The listing builds one solid part. Answer for the finished solid, in the listing's coordinates (mm). Round coordinates to 2 decimals unless told otherwise and drop trailing zeros. Write each loop counter-clockwise with the first axis right and the second up, starting at its lowest first coordinate (ties: lowest second). Pieces come first, ordered by that corner, then holes. Notation, with made-up numbers: (-31, 67) - (24, 67) arc R7 cw to (24, 71) - close; hole circle Ø6 at (-27, 74.25). An arc over 180 degrees is marked (long way). Answer in a Markdown table with one row per item.
from build123d import *

# Parameters (mm, degrees)
SKETCH1_W           = 210
SKETCH1_H           = 50
SKETCH1_R           = 1.211665018
SKETCH1_R_2         = 1.165617118
SKETCH1_R_3         = 1.5
SKETCH1_R_4         = 1.25
SKETCH1_R_5         = 1.517273905
BOSS_EXTRUDE1_DEPTH = 3.175
SKETCH2_R           = 2
CUT_EXTRUDE1_DEPTH  = 10
SKETCH3_R           = 6
SKETCH3_R_2         = 0.586995366
CUT_EXTRUDE2_DEPTH  = 57.15
CUT_EXTRUDE7_DEPTH  = 10
FILLET3_R           = 5
SKETCH11_R          = 18.5
SKETCH11_R_2        = 2
BOSS_EXTRUDE4_DEPTH = 3.175


with BuildPart() as part:
    # Sketch1 → Boss-Extrude1 (new body)
    with BuildSketch(Plane(origin=(0, 0, 0), x_dir=(1, 0, 0), z_dir=(0, 1, 0))):
        with Locations((105, -25)):
            Rectangle(SKETCH1_W, SKETCH1_H)
        with Locations(Location((3.489526233, -16.787661112, 0), (0, 0, 270))):
            Circle(SKETCH1_R, mode=Mode.SUBTRACT)
        with Locations(Location((34.37258772, -17.194005245, 0), (0, 0, 270))):
            Circle(SKETCH1_R_2, mode=Mode.SUBTRACT)
        with Locations(Location((37.520749958, -44.921198121, 0), (0, 0, 270))):
            Circle(SKETCH1_R_3, mode=Mode.SUBTRACT)
        with Locations(Location((118.879039361, -40.017685043, 0), (0, 0, 270))):
            Circle(SKETCH1_R_4, mode=Mode.SUBTRACT)
        with Locations(Location((112.302052499, -4.739260115, 0), (0, 0, 270))):
            Circle(SKETCH1_R_3, mode=Mode.SUBTRACT)
        with Locations(Location((168.975233936, -37.403209633, 0), (0, 0, 270))):
            Circle(SKETCH1_R_5, mode=Mode.SUBTRACT)
    extrude(amount=BOSS_EXTRUDE1_DEPTH)

    # Sketch2 → Cut-Extrude1 (cut)
    with BuildSketch(Plane(origin=(0, 3.175, 0), x_dir=(1, 0, 0), z_dir=(0, 1, 0))):
        with Locations(Location((10, -26, 0), (0, 0, 270))):
            Circle(SKETCH2_R)
        with Locations(Location((10, -42, 0), (0, 0, 270))):
            Circle(SKETCH2_R)
        with Locations(Location((26, -26, 0), (0, 0, 270))):
            Circle(SKETCH2_R)
        with Locations(Location((26, -42, 0), (0, 0, 270))):
            Circle(SKETCH2_R)
    extrude(amount=-CUT_EXTRUDE1_DEPTH, mode=Mode.SUBTRACT)

    # Sketch3 → Cut-Extrude2 (cut)
    with BuildSketch(Plane(origin=(0, 3.175, 0), x_dir=(1, 0, 0), z_dir=(0, 1, 0))):
        with Locations(Location((75.84991357, -28.1, 0), (0, 0, 270))):
            Circle(SKETCH3_R)
        with Locations(Location((140.771956051, -16, 0), (0, 0, 270))):
            Circle(SKETCH3_R)
        with Locations(Location((18, -34, 0), (0, 0, 270))):
            Circle(SKETCH3_R_2)
        with Locations(Location((197.921956051, -16, 0), (0, 0, 270))):
            Circle(SKETCH3_R)
    extrude(amount=-CUT_EXTRUDE2_DEPTH, mode=Mode.SUBTRACT)

    # Sketch10 → Cut-Extrude7 (cut)
    with BuildSketch(Plane(origin=(0, 3.175, 0), x_dir=(1, 0, 0), z_dir=(0, 1, 0))):
        Polygon((210, -27.859435908), (165.502877994, -50), (210, -50), align=None)
        Polygon((92.532613397, 0), (77.65477062, -7.402812063), (0, -7.402812063), (0, 0), align=None)
    extrude(amount=-CUT_EXTRUDE7_DEPTH, mode=Mode.SUBTRACT)

    # Fillet3
    fillet3_edges = [part.edges().sort_by_distance(p)[0] for p in [
        (210, 1.5875, 0),
        (0, 1.5875, 50),
        (92.532613397, 1.5875, 0),
        (210, 1.5875, 27.859435908),
        (165.502877994, 1.5875, 50),
        (77.65477062, 1.5875, 7.402812063),
        (0, 1.5875, 7.402812063),
    ]]
    fillet(fillet3_edges, radius=FILLET3_R)

    # Sketch11 → Boss-Extrude4 (add)
    with BuildSketch(Plane(origin=(0, 3.175, 0), x_dir=(1, 0, 0), z_dir=(0, 1, 0))):
        with Locations((18, -34)):
            Circle(SKETCH11_R)
        with Locations(Location((10, -26, 0), (0, 0, 270))):
            Circle(SKETCH11_R_2, mode=Mode.SUBTRACT)
        with Locations(Location((10, -42, 0), (0, 0, 270))):
            Circle(SKETCH11_R_2, mode=Mode.SUBTRACT)
        with Locations(Location((26, -26, 0), (0, 0, 270))):
            Circle(SKETCH11_R_2, mode=Mode.SUBTRACT)
        with Locations(Location((26, -42, 0), (0, 0, 270))):
            Circle(SKETCH11_R_2, mode=Mode.SUBTRACT)
    extrude(amount=-BOSS_EXTRUDE4_DEPTH)


solid = part.part
(1) For a pull along Z with two mould halves and no side action, classify faces 1 (the cylindrical face through (1.426, 1.565, 8.906)), 2 (the cylindrical face through (80.909, 1.61, 31.326)), 3 (the cylindrical face through (1, 2, 48)) as pulls with the +Z half, pulls with the -Z half, needs draft (parallel to the pull), parting line crosses it, or undercut.
Checked values:
| item | result |
|---|---|
| face 1 | pulls with the -Z half |
| face 2 | undercut |
| face 3 | pulls with the +Z half |
(2) Section A-A (y = 2.55) is taken. State how many separate pieces and enclosed holes the cut face has, and give its area (3 significant figures).
Checked values:
| item | result |
|---|---|
| separate pieces | 1 |
| enclosed holes | 13 |
| area | 8,970 mm2 |
(3) Section C-C (x = 66.5) is taken. Give the vertices of the cut face in (y, z) (3 decimals).
Checked values:
| item | result |
|---|---|
| outline | (0, 7.403) - (3.175, 7.403) - (3.175, 50) - (0, 50) - close |
(4) Section B-B (x = 149) is taken. Give the vertices of the cut face in (y, z) (3 decimals).
Checked values:
| item | result |
|---|---|
| outline | (0, 0) - (3.175, 0) - (3.175, 50) - (0, 50) - close |
(5) Find the intervals of material crossed by line 1 (X direction, y = 1.45, z = 42); line 2 (Z direction, x = 11.5, y = 0.65); line 3 (X direction, y = 1.15, z = 26), in increasing order.
Checked values:
| item | result |
|---|---|
| line 1 | x = 0 to 8, 12 to 24, 28 to 181.58 |
| line 2 | z = 7.4 to 24.68, 27.32 to 40.68, 43.32 to 51.32 |
| line 3 | x = 0 to 8, 12 to 24, 28 to 70.23, 81.47 to 209.84 |
(6) Flat-ended cylindrical pins translate along their axes: pin 1 (1.6 mm diameter, centred on x = 7, y = 1.5, fed in from +Z); pin 2 (7 mm diameter, centred on x = 75.85, z = 28.1, fed in from +Y). Find the tip coordinate at first contact, or state that the pin passes through.
Checked values:
| item | result |
|---|---|
| pin 1 | stops at z = 50 |
| pin 2 | passes through |
